Geometry check sheet. Reference: the model listing, model coordinates, mm. A direction names the side the tool comes from. Coordinates: 2 decimals unless noted, no trailing zeros. Order: outer loops, then holes, each group sorted by start corner. A loop starts at its lowest first (then second) coordinate and runs counter-clockwise, first axis right, second up. Notation, with made-up numbers: M -31.75,83.5 L -6.75,83.5 A12 ccw -6.75,94.5 Z; hole C 30,-14.75 d2. An arc over 180 degrees is marked long. Use CSV: the item, a comma, the result in double quotes. Start each with the question number.
```python
from build123d import *

# Parameters (mm, degrees)
ESQUISSE1_R             = 3.635
ESQUISSE1_R_2           = 1.2
BOSS_EXTRU_1_DEPTH      = 5.4
BOSS_EXTRU_2_DEPTH      = 1.95
ESQUISSE3_R             = 2.45
ENL_V_MAT_EXTRU_1_DEPTH = 1
ESQUISSE4_R             = 2.45
ENL_V_MAT_EXTRU_2_DEPTH = 3.7
ESQUISSE5_R             = 0.5
ENL_V_MAT_EXTRU_3_DEPTH = 3.7


with BuildPart() as part:
    # Esquisse1 → Boss.-Extru.1 (new body)
    with BuildSketch(Plane.XY):
        Circle(ESQUISSE1_R)
        Circle(ESQUISSE1_R_2, mode=Mode.SUBTRACT)
    extrude(amount=BOSS_EXTRU_1_DEPTH)

    # Esquisse2 → Boss.-Extru.2 (add)
    with BuildSketch(Plane.XY.offset(4.55)):
        with BuildLine():
            Line((2.224320121, 2.875), (14.344868259, 1.994746397))
            ThreePointArc((14.344868259, 1.994746397), (16.2, 0), (14.344868259, -1.994746397))
            Line((14.344868259, -1.994746397), (2.224320121, -2.875))
            ThreePointArc((2.224320121, -2.875), (3.635, 0), (2.224320121, 2.875))
        make_face()
    extrude(amount=-BOSS_EXTRU_2_DEPTH)

    # Esquisse3 → Enlèv. mat.-Extru.1 (cut)
    with BuildSketch(Plane.XY.offset(5.4)):
        Circle(ESQUISSE3_R)
    extrude(amount=-ENL_V_MAT_EXTRU_1_DEPTH, mode=Mode.SUBTRACT)

    # Esquisse4 → Enlèv. mat.-Extru.2 (cut)
    with BuildSketch(Plane(origin=(0, 0, 0), x_dir=(-1, 0, 0), z_dir=(0, 0, -1))):
        Circle(ESQUISSE4_R)
    extrude(amount=-ENL_V_MAT_EXTRU_2_DEPTH, mode=Mode.SUBTRACT)

    # Esquisse5 → Enlèv. mat.-Extru.3 (cut)
    with BuildSketch(Plane.XY.offset(4.55)):
        with Locations((14.7, 0)):
            Circle(ESQUISSE5_R)
        with Locations((12.7, 0)):
            Circle(ESQUISSE5_R)
        with Locations((10.7, 0)):
            Circle(ESQUISSE5_R)
        with Locations((8.7, 0)):
            Circle(ESQUISSE5_R)
        with Locations((6.7, 0)):
            Circle(ESQUISSE5_R)
        with Locations((4.7, 0)):
            Circle(ESQUISSE5_R)
    extrude(amount=-ENL_V_MAT_EXTRU_3_DEPTH, mode=Mode.SUBTRACT)


solid = part.part
```
1) Material ranges on line 1 along Y through (x, z) = (0, 2.1) (3 decimals); line 2 along Z through (x, y) = (6.75, -1); line 3 along Z through (x, y) = (0.75, 2), recorded low to high.
2) Section check C-C on y = 0.75. Record the boundary of the cut face in (x, z).
3) Section check B-B on z = 3.05. Record the boundary of the cut face in (x, y) (3 decimals), then the cut area to 3 significant figures.
4) Set-up check for faces 4 (the face through (15.177, 0.15, 3.589)), 5 (the face through (0.5, -2.4, 1.8)), 6 (the face through (-0.5, -2.4, 4.9)): record each of +Z, -Z, +X, -X, +Y, -Y from which the full face is reachable in a straight line by a thin tool's end or side.
5) Draft check along Y on faces 1 (the face through (-1, 1, 3.7)), 2 (the face through (9, -1, 2.6)), 3 (the face through (16.2, 0, 3.6)). Enter one of: +Y half, -Y half, draft (parallel to the pull), parting line (faces both ways), or undercut.
6) Gauge pin test, flat ends, axial feed: P1, Ø1.7, axis at x = 12, y = 1, coming from the +Z side; P2, Ø1.5, axis at x = -1, y = 1, coming from the -Z side; P3, Ø1.7, axis at x = 7, y = 1.5, coming from the -Z side. Record the tip position at first contact, or that the pin passes through.
7) Section check A-A on x = 0. Record the boundary of the cut face in (y, z) (3 decimals), then the cut area to 3 significant figures.
8) Section check D-D on x = -2. Record the boundary of the cut face in (y, z), then the cut area to 3 significant figures.
Results are:
1,line 1,"y = -3.635 to -2.45, 2.45 to 3.635"
1,line 2,"z = 2.6 to 4.55"
1,line 3,"z = 3.7 to 4.4"
2,outline,"M -3.56,0 L -2.33,0 L -2.33,3.7 L -0.94,3.7 L -0.94,4.4 L -2.33,4.4 L -2.33,5.4 L -3.56,5.4 Z; M 0.94,3.7 L 2.33,3.7 L 2.33,0 L 3.56,0 L 3.56,2.6 L 16.05,2.6 L 16.05,4.55 L 3.56,4.55 L 3.56,5.4 L 2.33,5.4 L 2.33,4.4 L 0.94,4.4 Z"
3,outline,"M 2.224,-2.875 L 14.345,-1.995 A2 ccw 14.345,1.995 L 2.224,2.875 A3.635 ccw long Z; hole C 0,0 d4.9; hole C 4.7,0 d1; hole C 6.7,0 d1; hole C 8.7,0 d1; hole C 10.7,0 d1; hole C 12.7,0 d1; hole C 14.7,0 d1"
3,area,"77.0 mm²"
4,face 4,"+Z, -Z"
4,face 5,"-Z"
4,face 6,"+Z"
5,face 1,"undercut"
5,face 2,"draft"
5,face 3,"parting line"
6,P1,"stops at z = 4.55"
6,P2,"stops at z = 3.7"
6,P3,"stops at z = 2.6"
7,outline,"M -3.635,0 L -2.45,0 L -2.45,3.7 L -1.2,3.7 L -1.2,4.4 L -2.45,4.4 L -2.45,5.4 L -3.635,5.4 Z; M 1.2,3.7 L 2.45,3.7 L 2.45,0 L 3.635,0 L 3.635,5.4 L 2.45,5.4 L 2.45,4.4 L 1.2,4.4 Z"
7,area,"14.5 mm²"
8,outline,"M -3.04,0 L -1.42,0 L -1.42,3.7 L 1.42,3.7 L 1.42,0 L 3.04,0 L 3.04,5.4 L 1.42,5.4 L 1.42,4.4 L -1.42,4.4 L -1.42,5.4 L -3.04,5.4 Z"
8,area,"19.5 mm²"
